For this review, take the finished solid that the model builds, in its own axes (mm). Coordinates: 2 decimals unless noted, no trailing zeros. Write each loop counter-clockwise with the first axis right and the second up, starting at its lowest first coordinate (ties: lowest second). Pieces come first, ordered by that corner, then holes. Notation, with made-up numbers: (30, 76.25) -> (39, 76.25) arc R7 cw to (39, 88.25) -> close; hole circle Ø10 at (69, 4.25). An arc over 180 degrees is marked (long way). Put each result on its own line as item: value. Start each with the question number.
Item 1: Consider section D-D on y = 1.8. Give the boundary of the cut face in (x, z) (3 decimals).
Item 2: Insertion check: P1, Ø0.6, axis at x = 9, z = -10, coming from the +Y side; P2, Ø1.5, axis at x = -7.5, z = 0, coming from the -Y side; P3, Ø0.7, axis at x = -11.5, y = 1, coming from the -Z side; P4, Ø1, axis at x = -15, z = 10, coming from the +Y side. Each pin has a flat end and moves straight along its axis. Give the tip position at first contact, or say it passes through.
Item 3: Consider section C-C on x = 14.5. Give the boundary of the cut face in (y, z) (3 decimals), and give its area (3 significant figures).
Item 4: Consider section A-A on x = -16. Give the boundary of the cut face in (y, z) (3 decimals), and give its area (3 significant figures).
Item 5: To check wall thickness, follow L1, parallel to X at y = 1.85, z = -6 (3 decimals); L2, parallel to Y at x = 14, z = 3.5; L3, parallel to Y at x = 8.5, z = 3.75. State the ranges of each line that lie inside material, in increasing order.
```python
from build123d import *

# Parameters (mm, degrees)
SKETCH_1_W      = 16.51
SKETCH_1_H      = 22.86
EXTRUDE_1_DEPTH = 3.18
CHAMFER_1_SIZE  = 1
CHAMFER_1_SIZE2 = 2.475086853
SKETCH_2_W      = 3.305
SKETCH_2_H      = 0.15
SKETCH_2_W_2    = 5.59
SKETCH_4_W      = 3.3
SKETCH_4_H      = 0.15
SKETCH_4_W_2    = 4.575
CHAMFER_2_SIZE  = 2


with BuildPart() as part:
    # Эскиз1 → Бобышка-Вытянуть1 (new body)
    with BuildSketch(Plane(origin=(0, 0, 0), x_dir=(1, 0, 0), z_dir=(0, 1, 0))):
        Rectangle(SKETCH_1_W, SKETCH_1_H)
    extrude(amount=EXTRUDE_1_DEPTH)

    # Фаска1
    chamfer_1_edges = [part.edges().sort_by_distance(p)[0] for p in [
        (-8.255, 3.18, 0),
    ]]
    chamfer_1_side = [part.faces().sort_by_distance(p)[0] for p in [
        (-8.255, 1.59, 0),
    ]]
    chamfer(chamfer_1_edges, length=CHAMFER_1_SIZE, length2=CHAMFER_1_SIZE2, reference=chamfer_1_side[0])

    # По траектории1: sweep along a path in Эскиз3
    with BuildLine(Plane.XY) as sweep_1_path:
        Line((18.415, 0), (11.196173743, 0))
        ThreePointArc((11.196173743, 0), (10.877975692, 0.131801948), (10.746173743, 0.45))
        Line((10.746173743, 0.45), (10.746173743, 0.79))
        ThreePointArc((10.746173743, 0.79), (10.614371795, 1.108198052), (10.296173743, 1.24))
        Line((10.296173743, 1.24), (8.255, 1.24))
    # Эскиз2 → По траектории1 (sweep)
    with BuildSketch(Plane(origin=(8.255, 0, 0), x_dir=(0, 0, -1), z_dir=(1, 0, 0))):
        with Locations((-9.2725, 1.315)):
            Rectangle(SKETCH_2_W, SKETCH_2_H)
        with Locations((-3.555, 1.315)):
            Rectangle(SKETCH_2_W_2, SKETCH_2_H)
        with Locations((3.555, 1.315)):
            Rectangle(SKETCH_2_W_2, SKETCH_2_H)
        with Locations((9.2725, 1.315)):
            Rectangle(SKETCH_2_W, SKETCH_2_H)
    sweep(path=sweep_1_path.line)

    # По траектории2: sweep along a path in Эскиз5
    with BuildLine(Plane.XY) as sweep_2_path:
        Line((-8.255, 1.24), (-10.296173743, 1.24))
        ThreePointArc((-10.296173743, 1.24), (-10.614371795, 1.108198052), (-10.746173743, 0.79))
        Line((-10.746173743, 0.79), (-10.746173743, 0.45))
        ThreePointArc((-10.746173743, 0.45), (-10.877975692, 0.131801948), (-11.196173743, 0))
        Line((-11.196173743, 0), (-18.415, 0))
    # Эскиз4 → По траектории2 (sweep)
    with BuildSketch(Plane.ZY.offset(8.255)):
        with Locations((-9.275, 1.315)):
            Rectangle(SKETCH_4_W, SKETCH_4_H)
        with Locations((-3.5575, 1.315)):
            Rectangle(SKETCH_4_W_2, SKETCH_4_H)
        with Locations((3.5575, 1.315)):
            Rectangle(SKETCH_4_W_2, SKETCH_4_H)
        with Locations((9.275, 1.315)):
            Rectangle(SKETCH_4_W, SKETCH_4_H)
    sweep(path=sweep_2_path.line)

    # Фаска2
    chamfer_2_edges = [part.edges().sort_by_distance(p)[0] for p in [
        (18.415, 0.075, 0.76),
        (18.415, 0.075, -6.35),
    ]]
    chamfer(chamfer_2_edges, length=CHAMFER_2_SIZE)


solid = part.part
```
Return value:
1. outline: (-8.255, -11.43) -> (8.255, -11.43) -> (8.255, 11.43) -> (-8.255, 11.43) -> close
2. P1: y = 1.39
2. P2: y = 0
2. P3: through
2. P4: y = 0.15
3. outline: (0, -10.925) -> (0.15, -10.925) -> (0.15, -7.62) -> (0, -7.62) -> close; (0, -6.35) -> (0.15, -6.35) -> (0.15, -0.76) -> (0, -0.76) -> close; (0, 0.76) -> (0.15, 0.76) -> (0.15, 6.35) -> (0, 6.35) -> close; (0, 7.62) -> (0.15, 7.62) -> (0.15, 10.925) -> (0, 10.925) -> close
3. area: 2.67 mm^2
4. outline: (0, -10.925) -> (0.15, -10.925) -> (0.15, -7.625) -> (0, -7.625) -> close; (0, -5.845) -> (0.15, -5.845) -> (0.15, -1.27) -> (0, -1.27) -> close; (0, 1.27) -> (0.15, 1.27) -> (0.15, 5.845) -> (0, 5.845) -> close; (0, 7.625) -> (0.15, 7.625) -> (0.15, 10.925) -> (0, 10.925) -> close
4. area: 2.36 mm^2
5. L1: -8.255 to 8.255
5. L2: 0 to 0.15
5. L3: 1.24 to 1.39
